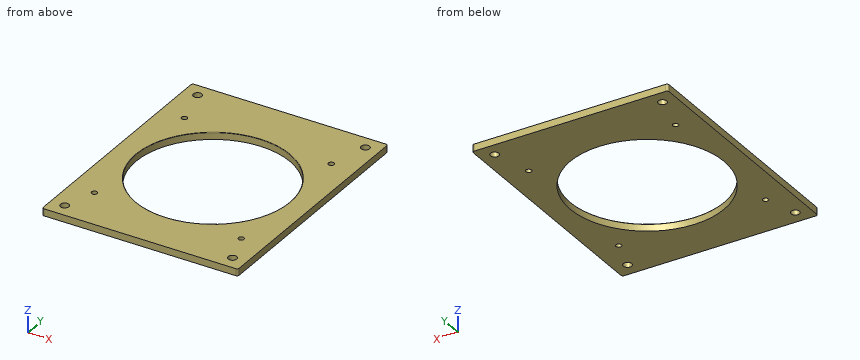
from build123d import *

# Parameters (mm, degrees)
BOSS_EXTRU_1_DEPTH      = 5
ESQUISSE4_R             = 3
ENL_V_MAT_EXTRU_3_DEPTH = 10
ESQUISSE5_R             = 2
ESQUISSE5_R_2           = 55
ENL_V_MAT_EXTRU_4_DEPTH = 10
CONG_1_R                = 0.25


with BuildPart() as part:
    # Esquisse1 → Boss.-Extru.1 (new body)
    with BuildSketch(Plane.XY):
        with BuildLine():
            Line((-68, 87.5), (-68.5, 87.5))
            ThreePointArc((-68.5, 87.5), (-69.560660172, 87.060660172), (-70, 86))
            Line((-70, 86), (-70, 75.5))
            Line((-70, 75.5), (-70, -85.5))
            Line((-70, -85.5), (-70, -86))
            ThreePointArc((-70, -86), (-69.560660172, -87.060660172), (-68.5, -87.5))
            Line((-68.5, -87.5), (-68, -87.5))
            Line((-68, -87.5), (68, -87.5))
            Line((68, -87.5), (68.5, -87.5))
            ThreePointArc((68.5, -87.5), (69.560660172, -87.060660172), (70, -86))
            Line((70, -86), (70, -85.5))
            Line((70, -85.5), (70, 75.5))
            Line((70, 75.5), (70, 86))
            ThreePointArc((70, 86), (69.560660172, 87.060660172), (68.5, 87.5))
            Line((68.5, 87.5), (68, 87.5))
            Line((68, 87.5), (-68, 87.5))
        make_face()
    extrude(amount=BOSS_EXTRU_1_DEPTH)

    # Esquisse4 → Enlèv. mat.-Extru.3 (cut)
    with BuildSketch(Plane.XY.offset(5)):
        with Locations((-60, -77.5)):
            Circle(ESQUISSE4_R)
        with Locations((60, -77.5)):
            Circle(ESQUISSE4_R)
        with Locations((-60, 77.5)):
            Circle(ESQUISSE4_R)
        with Locations((60, 77.5)):
            Circle(ESQUISSE4_R)
    extrude(amount=-ENL_V_MAT_EXTRU_3_DEPTH, mode=Mode.SUBTRACT)

    # Esquisse5 → Enlèv. mat.-Extru.4 (cut)
    with BuildSketch(Plane(origin=(0, 0, 0), x_dir=(-1, 0, 0), z_dir=(0, 0, -1))):
        with Locations((-52.5, 50)):
            Circle(ESQUISSE5_R)
        with Locations((52.5, 50)):
            Circle(ESQUISSE5_R)
        with Locations((52.5, -55)):
            Circle(ESQUISSE5_R)
        with Locations((-52.5, -55)):
            Circle(ESQUISSE5_R)
        with Locations((0, -2.5)):
            Circle(ESQUISSE5_R_2)
    extrude(amount=-ENL_V_MAT_EXTRU_4_DEPTH, mode=Mode.SUBTRACT)

    # Congé1
    cong_1_edges = [part.edges().sort_by_distance(p)[0] for p in [
        (55, -2.5, 5),
    ]]
    fillet(cong_1_edges, radius=CONG_1_R)


solid = part.part
Verification items for the finished model (mm, model axes). Coordinates: 2 decimals unless noted, no trailing zeros. Order: outer loops, then holes, each group sorted by start corner. A loop starts at its lowest first (then second) coordinate and runs counter-clockwise, first axis right, second up. Notation, with made-up numbers: M 84.25,13.5 L 124.25,13.5 A25 cw 124.25,42.5 Z; hole C 15.25,67 d5. An arc over 180 degrees is marked long. One line per item, written item: value. Start each with the question number.
Item 1: Sectioned sample at B-B on y = -77.5. Record the cut outline in (x, z), then the cut area to 3 significant figures.
Item 2: Depth check by flat-ended pin: P1, Ø5, axis at x = -52.5, y = 50, coming from the -Z side. Enter the tip coordinate at first touch or a pass-through.
Item 3: Thickness scan on probe 1 along Y at (x, z) = (-60, 2.55); probe 2 along X at (y, z) = (76, 1.7); probe 3 along Y at (x, z) = (14, 1.2). Record the ranges inside material, lowest first.
Item 4: Sectioned sample at C-C on x = 60. Record the cut outline in (y, z).
Item 5: Sectioned sample at A-A on z = 1.45. Give the number of separate pieces and of enclosed holes in the cut face, then the cut area to 3 significant figures.
Calculated:
1. outline: M -70,0 L -63,0 L -63,5 L -70,5 Z; M -57,0 L 57,0 L 57,5 L -57,5 Z; M 63,0 L 70,0 L 70,5 L 63,5 Z
1. area: 640 mm^2
2. P1: z = 0
3. probe 1: -87.5 to -80.5, -74.5 to 74.5, 80.5 to 87.5
3. probe 2: -70 to -62.6, -57.4 to 57.4, 62.6 to 70
3. probe 3: -87.5 to -55.69, 50.69 to 87.5
4. outline: M -87.5,0 L -80.5,0 L -80.5,5 L -87.5,5 Z; M -74.5,0 L 74.5,0 L 74.5,5 L -74.5,5 Z; M 80.5,0 L 87.5,0 L 87.5,5 L 80.5,5 Z
5. separate pieces: 1
5. enclosed holes: 9
5. area: 14,800 mm^2
